from build123d import *

# Parameters (mm, degrees)
SKETCH1_R           = 137.5
BOSS_EXTRUDE1_DEPTH = 1.2
SKETCH3_R           = 2.25
CUT_EXTRUDE1_DEPTH  = 2.2
CUT_EXTRUDE2_DEPTH  = 1.2
SKETCH5_R           = 1.5
CUT_EXTRUDE3_DEPTH  = 2.2
SKETCH6_R           = 1.5
CUT_EXTRUDE4_DEPTH  = 2.2
SKETCH7_W           = 5
SKETCH7_H           = 3
CUT_EXTRUDE5_DEPTH  = 2.2


with BuildPart() as part:
    # Sketch1 → Boss-Extrude1 (new body)
    with BuildSketch(Plane(origin=(0, 0, 0), x_dir=(1, 0, 0), z_dir=(0, 1, 0))):
        Circle(SKETCH1_R)
    extrude(amount=BOSS_EXTRUDE1_DEPTH)

    # Sketch3 → Cut-Extrude1 (cut, through all)
    with BuildSketch(Plane(origin=(0, 1.2, 0), x_dir=(1, 0, 0), z_dir=(0, 1, 0))):
        with Locations((0, 127.454948432)):
            Circle(SKETCH3_R)
        with Locations((19.938346675, 125.885766517)):
            Circle(SKETCH3_R)
        with Locations((39.385745083, 121.21685924)):
            Circle(SKETCH3_R)
        with Locations((57.863335733, 113.563190593)):
            Circle(SKETCH3_R)
        with Locations((74.91613902, 103.113219299)):
            Circle(SKETCH3_R)
        with Locations((90.124258332, 90.124258332)):
            Circle(SKETCH3_R)
        with Locations((103.113219299, 74.91613902)):
            Circle(SKETCH3_R)
        with Locations((113.563190593, 57.863335733)):
            Circle(SKETCH3_R)
        with Locations((121.21685924, 39.385745083)):
            Circle(SKETCH3_R)
        with Locations((125.885766517, 19.938346675)):
            Circle(SKETCH3_R)
        with Locations((127.454948432, 0)):
            Circle(SKETCH3_R)
        with Locations((125.885766517, -19.938346675)):
            Circle(SKETCH3_R)
        with Locations((121.21685924, -39.385745083)):
            Circle(SKETCH3_R)
        with Locations((113.563190593, -57.863335733)):
            Circle(SKETCH3_R)
        with Locations((103.113219299, -74.91613902)):
            Circle(SKETCH3_R)
        with Locations((90.124258332, -90.124258332)):
            Circle(SKETCH3_R)
        with Locations((74.91613902, -103.113219299)):
            Circle(SKETCH3_R)
        with Locations((57.863335733, -113.563190593)):
            Circle(SKETCH3_R)
        with Locations((39.385745083, -121.21685924)):
            Circle(SKETCH3_R)
        with Locations((19.938346675, -125.885766517)):
            Circle(SKETCH3_R)
        with Locations((0, -127.454948432)):
            Circle(SKETCH3_R)
        with Locations((-19.938346675, -125.885766517)):
            Circle(SKETCH3_R)
        with Locations((-39.385745083, -121.21685924)):
            Circle(SKETCH3_R)
        with Locations((-57.863335733, -113.563190593)):
            Circle(SKETCH3_R)
        with Locations((-74.91613902, -103.113219299)):
            Circle(SKETCH3_R)
        with Locations((-90.124258332, -90.124258332)):
            Circle(SKETCH3_R)
        with Locations((-103.113219299, -74.91613902)):
            Circle(SKETCH3_R)
        with Locations((-113.563190593, -57.863335733)):
            Circle(SKETCH3_R)
        with Locations((-121.21685924, -39.385745083)):
            Circle(SKETCH3_R)
        with Locations((-125.885766517, -19.938346675)):
            Circle(SKETCH3_R)
        with Locations((-127.454948432, 0)):
            Circle(SKETCH3_R)
        with Locations((-125.885766517, 19.938346675)):
            Circle(SKETCH3_R)
        with Locations((-121.21685924, 39.385745083)):
            Circle(SKETCH3_R)
        with Locations((-113.563190593, 57.863335733)):
            Circle(SKETCH3_R)
        with Locations((-103.113219299, 74.91613902)):
            Circle(SKETCH3_R)
        with Locations((-90.124258332, 90.124258332)):
            Circle(SKETCH3_R)
        with Locations((-74.91613902, 103.113219299)):
            Circle(SKETCH3_R)
        with Locations((-57.863335733, 113.563190593)):
            Circle(SKETCH3_R)
        with Locations((-39.385745083, 121.21685924)):
            Circle(SKETCH3_R)
        with Locations((-19.938346675, 125.885766517)):
            Circle(SKETCH3_R)
    extrude(amount=-CUT_EXTRUDE1_DEPTH, mode=Mode.SUBTRACT)

    # Sketch4 → Cut-Extrude2 (cut)
    with BuildSketch(Plane(origin=(0, 1.2, 0), x_dir=(1, 0, 0), z_dir=(0, 1, 0))):
        Polygon((-107.5, -43), (-107.5, 43), (-105.5, 45), (-94.5, 45), (-92.5, 43), (-92.5, 9.5), (-91, 9.5), (-91, 11.5), (-77, 11.5), (-77, 5.5), (-67, 5.5), (-67, 11.5), (-44, 11.5), (-42, 9.5), (-42, -9.5), (-44, -11.5), (-67, -11.5), (-67, -5.5), (-77, -5.5), (-77, -11.5), (-91, -11.5), (-91, -9.5), (-92.5, -9.5), (-92.5, -43), (-94.5, -45), (-105.5, -45), align=None)
        Polygon((94.5, -45), (92.5, -43), (92.5, -9.5), (91, -9.5), (91, -11.5), (77, -11.5), (77, -5.5), (67, -5.5), (67, -11.5), (44, -11.5), (42, -9.5), (42, 9.5), (44, 11.5), (67, 11.5), (67, 5.5), (77, 5.5), (77, 11.5), (91, 11.5), (91, 9.5), (92.5, 9.5), (92.5, 43), (94.5, 45), (105.5, 45), (107.5, 43), (107.5, -43), (105.5, -45), align=None)
    extrude(amount=-CUT_EXTRUDE2_DEPTH, mode=Mode.SUBTRACT)

    # Sketch5 → Cut-Extrude3 (cut, through all)
    with BuildSketch(Plane(origin=(0, 1.2, 0), x_dir=(1, 0, 0), z_dir=(0, 1, 0))):
        with Locations((-53.4, 84)):
            Circle(SKETCH5_R)
        with Locations((53.4, 84)):
            Circle(SKETCH5_R)
        with Locations((53.4, -24)):
            Circle(SKETCH5_R)
        with Locations((-53.4, -24)):
            Circle(SKETCH5_R)
    extrude(amount=-CUT_EXTRUDE3_DEPTH, mode=Mode.SUBTRACT)

    # Sketch6 → Cut-Extrude4 (cut, through all)
    with BuildSketch(Plane(origin=(0, 1.2, 0), x_dir=(1, 0, 0), z_dir=(0, 1, 0))):
        with Locations((-12.5, 110)):
            Circle(SKETCH6_R)
        with Locations((12.5, 110)):
            Circle(SKETCH6_R)
        with Locations((12.5, 85)):
            Circle(SKETCH6_R)
        with Locations((-12.5, 85)):
            Circle(SKETCH6_R)
        with Locations((-12.5, -85)):
            Circle(SKETCH6_R)
        with Locations((12.5, -85)):
            Circle(SKETCH6_R)
        with Locations((12.5, -110)):
            Circle(SKETCH6_R)
        with Locations((-12.5, -110)):
            Circle(SKETCH6_R)
    extrude(amount=-CUT_EXTRUDE4_DEPTH, mode=Mode.SUBTRACT)

    # Sketch7 → Cut-Extrude5 (cut, through all)
    with BuildSketch(Plane(origin=(0, 1.2, 0), x_dir=(1, 0, 0), z_dir=(0, 1, 0))):
        with Locations((-72, 15.5)):
            Rectangle(SKETCH7_W, SKETCH7_H)
        with Locations((-72, -15.5)):
            Rectangle(SKETCH7_W, SKETCH7_H)
        with Locations((72, -15.5)):
            Rectangle(SKETCH7_W, SKETCH7_H)
        with Locations((72, 15.5)):
            Rectangle(SKETCH7_W, SKETCH7_H)
    extrude(amount=-CUT_EXTRUDE5_DEPTH, mode=Mode.SUBTRACT)


solid = part.part
The listing builds one solid part. Answer for the finished solid, in the listing's coordinates (mm). Coordinates: 2 decimals unless noted, no trailing zeros. Loops run counter-clockwise (first coordinate to the right, second up) from the corner with the lowest first, then second, coordinate; pieces in that order, holes last.
1) Find section A-A on x = 83. Write down the section's boundary in (y, z), then the cut area to 3 significant figures.
2) Find section B-B on x = 33.5. Write down the section's boundary in (y, z), then the cut area to 3 significant figures.
3) Flat-ended cylindrical pins translate along their axes: pin 1 Ø3.5 at (x, z) = (90.12, 90.12) entering from +Y; pin 2 Ø0.6 at (x, y) = (-54.5, 1) entering from +Z; pin 3 Ø0.6 at (x, y) = (54, 0.5) entering from +Z. Find the tip coordinate at first contact, or state that the pin passes through.
4) Find section C-C on y = 0.8. Give the number of separate pieces and of enclosed holes in the cut face, then the cut area to 3 significant figures.
5) Find the intervals of material crossed by L1, parallel to X at y = 1.15, z = -30; L2, parallel to Z at x = 75.5, y = 0.8; L3, parallel to Z at x = -122.5, y = 0.85, in increasing order.
Values:
1. outline: (0, -109.62) - (1.2, -109.62) - (1.2, -11.5) - (0, -11.5) - close; (0, 11.5) - (1.2, 11.5) - (1.2, 109.62) - (0, 109.62) - close
1. area: 235 mm2
2. outline: (0, -133.36) - (1.2, -133.36) - (1.2, 133.36) - (0, 133.36) - close
2. area: 320 mm2
3. pin 1: passes through
3. pin 2: stops at z = 126.37
3. pin 3: stops at z = 126.58
4. separate pieces: 1
4. enclosed holes: 58
4. area: 53,900 mm2
5. L1: x = -134.19 to -107.5, -92.5 to 92.5, 107.5 to 134.19
5. L2: z = -114.92 to -105.29, -100.94 to -5.5, 5.5 to 100.94, 105.29 to 114.92
5. L3: z = -62.45 to -41.23, -37.54 to 37.54, 41.23 to 62.45
